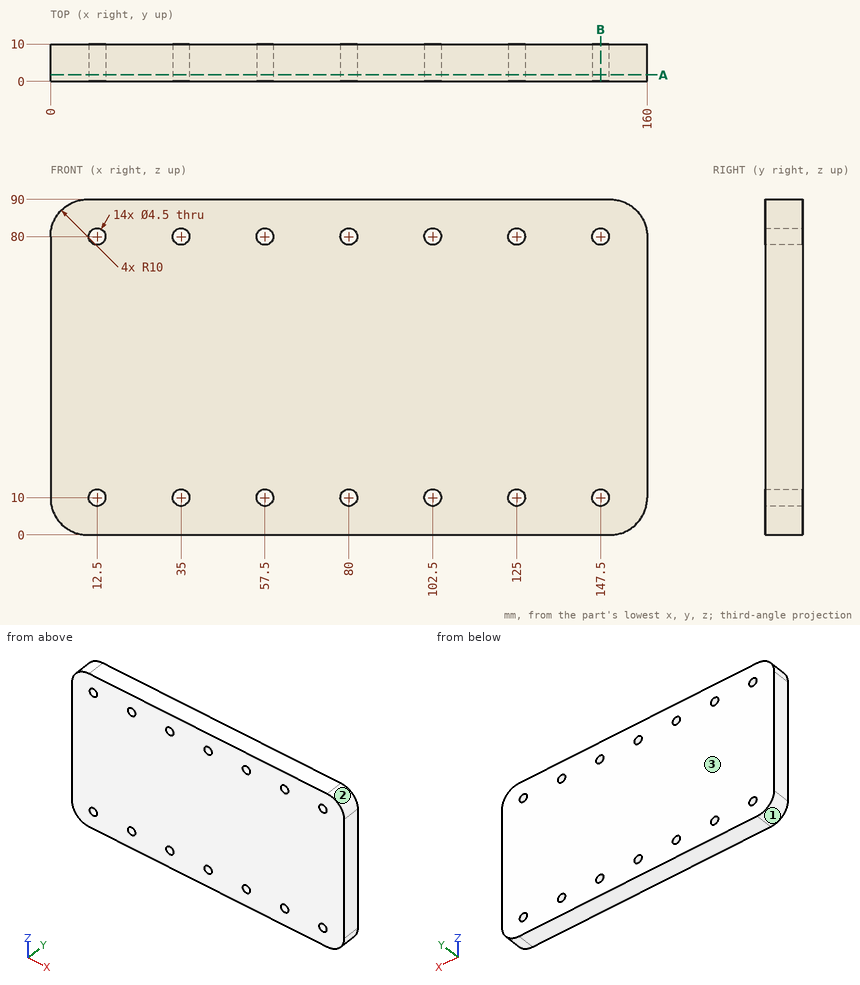
Could you check a few things on this drawing? It's one solid part, dimensions in mm from its lowest x, y, z. Coordinates: 2 decimals unless noted, no trailing zeros. Write each loop counter-clockwise with the first axis right and the second up, starting at its lowest first coordinate (ties: lowest second). Pieces come first, ordered by that corner, then holes. Notation, with made-up numbers: (75, -8) - (132, -8) arc R10 ccw to (132, 1) - close; hole circle Ø11 at (24.25, -18.5). An arc over 180 degrees is marked (long way). Write item = value, one per line.
1) We'd pull the mould along X, two halves only. Please class the marked faces 1, 2 and 3: +X half, -X half, draft (parallel to the pull), parting line (faces both ways), or undercut.
Result set:
face_1 = -X half
face_2 = +X half
face_3 = draft
2) Suppose I cut it at A-A on y = 1.75. State how many separate pieces and enclosed holes the cut face has, plus the area to 3 significant figures.
Result set:
separate_pieces = 1
enclosed_holes = 14
area = 14,100 mm2
3) Suppose I cut it at B-B on x = 147.5. Please give me the cut outline in (y, z), plus the area to 3 significant figures.
Result set:
outline = (0, 0) - (10, 0) - (10, 7.75) - (0, 7.75) - close; (0, 12.25) - (10, 12.25) - (10, 77.75) - (0, 77.75) - close; (0, 82.25) - (10, 82.25) - (10, 90) - (0, 90) - close
area = 810 mm2
4) Please list where these lines run through material, in increasing order: line 1 (Z direction, x = 147.5, y = 3.25); line 2 (Z direction, x = 82, y = 6.5); line 3 (X direction, y = 5, z = 7.5). Write a range as [from, to].
Result set:
line_1 = [0, 7.75], [12.25, 77.75], [82.25, 90]
line_2 = [0, 8.97], [11.03, 78.97], [81.03, 90]
line_3 = [0.32, 159.68]
5) Will this pin go through, and if not, where does the flat tip stop? pin 1 Ø7 at (x, z) = (147.5, 80) entering from -Y.
Result set:
pin_1 = 0
